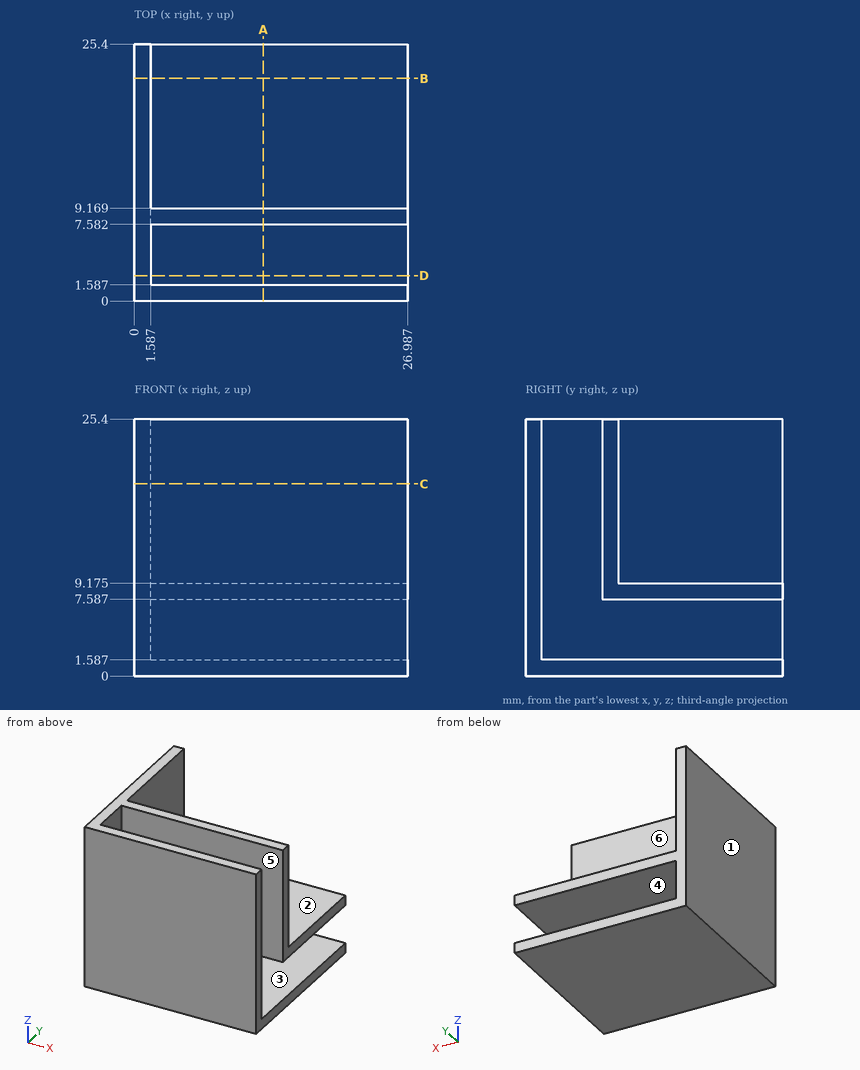
Could you check a few things on this drawing? It's one solid part, dimensions in mm from its lowest x, y, z. A direction names the side the tool comes from. Give positions to 0.01 mm unless a question says otherwise; leave off trailing zeros. Order: outer loops, then holes, each group sorted by start corner. A loop starts at its lowest first (then second) coordinate and runs counter-clockwise, first axis right, second up. Notation, with made-up numbers: (21.5, 79.5) - (40.5, 79.5) arc R34 cw to (40.5, 111.5) - close; hole circle Ø7 at (39.5, 9.25). An arc over 180 degrees is marked (long way). Return JSON: item names as keys, results as strings. Group by question number.
Q1. Suppose I cut it at A-A, the plane x = 12.75. Please give me the cut outline in (y, z) (1 decimal), and give its area (3 significant figures).
Q2. Thinking about a two-plate mould opening in Y: for the marked faces 4, 5 and 6, which applies, pulls with the +Y half, pulls with the -Y half, needs draft (parallel to the pull), parting line crosses it, or undercut?
Q3. Which directions (+Z, -Z, +X, -X, +Y, -Y) give clear straight access to the entire face, cutting with the end or side of a thin tool? Please do the marked faces 1, 2 and 3.
Q4. Will these pins go through, and if not, where does the flat tip stop? pin 1 Ø4 at (x, z) = (22, 13.5) entering from +Y; pin 2 Ø1 at (y, z) = (22.5, 18.5) entering from +X; pin 3 Ø8 at (x, y) = (16, 19) entering from +Z (1 decimal).
Q5. Suppose I cut it at D-D, the plane y = 2.5. Please give me the cut outline in (x, z).
Q6. Suppose I cut it at B-B, the plane y = 22. Please give me the cut outline in (x, z) (1 decimal), and give its area (3 significant figures).
Q7. Suppose I cut it at C-C, the plane z = 19. Please give me the cut outline in (x, y).
Q8. Please list where these lines run through material, in increasing order: line 1 along Z through (x, y) = (3.25, 14.25) (1 decimal); line 2 along Y through (x, z) = (4.5, 21.75); line 3 along Z through (x, y) = (4, 6.5). Write a range as [from, to].
Resolved:
{
 "1": {"outline": "(0, 0) - (25.4, 0) - (25.4, 1.6) - (1.6, 1.6) - (1.6, 25.4) - (0, 25.4) - close; (7.6, 7.6) - (25.4, 7.6) - (25.4, 9.2) - (9.2, 9.2) - (9.2, 25.4) - (7.6, 25.4) - close", "area": "132 mm2"},
 "2": {"face 4": "needs draft", "face 5": "undercut", "face 6": "pulls with the +Y half"},
 "3": {"face 1": "+Z, -Z, -X, +Y, -Y", "face 2": "+Z, +X, +Y", "face 3": "+X, +Y"},
 "4": {"pin 1": "stops at y = 9.17", "pin 2": "stops at x = 1.59", "pin 3": "stops at z = 9.2"},
 "5": {"outline": "(0, 0) - (26.99, 0) - (26.99, 1.59) - (1.59, 1.59) - (1.59, 25.4) - (0, 25.4) - close"},
 "6": {"outline": "(0, 0) - (27, 0) - (27, 1.6) - (1.6, 1.6) - (1.6, 7.6) - (27, 7.6) - (27, 9.2) - (1.6, 9.2) - (1.6, 25.4) - (0, 25.4) - close", "area": "121 mm2"},
 "7": {"outline": "(0, 0) - (26.99, 0) - (26.99, 1.59) - (1.59, 1.59) - (1.59, 7.58) - (26.99, 7.58) - (26.99, 9.17) - (1.59, 9.17) - (1.59, 25.4) - (0, 25.4) - close"},
 "8": {"line 1": "z = [0, 1.6], [7.6, 9.2]", "line 2": "y = [0, 1.59], [7.58, 9.17]", "line 3": "z = [0, 1.59]"}
}
